Geometry check sheet. Reference: drawing and pictorial views, mm from the part's lowest x, y, z. A direction names the side the tool comes from. Coordinates: 2 decimals unless noted, no trailing zeros. Loops run counter-clockwise (first coordinate to the right, second up) from the corner with the lowest first, then second, coordinate; pieces in that order, holes last. Notation, with made-up numbers: (-10, 54.5) - (46, 54.5) arc R14 cw to (46, 78.5) - close; hole circle Ø2 at (54.5, 67). An arc over 180 degrees is marked (long way). One line per item, written item: value.
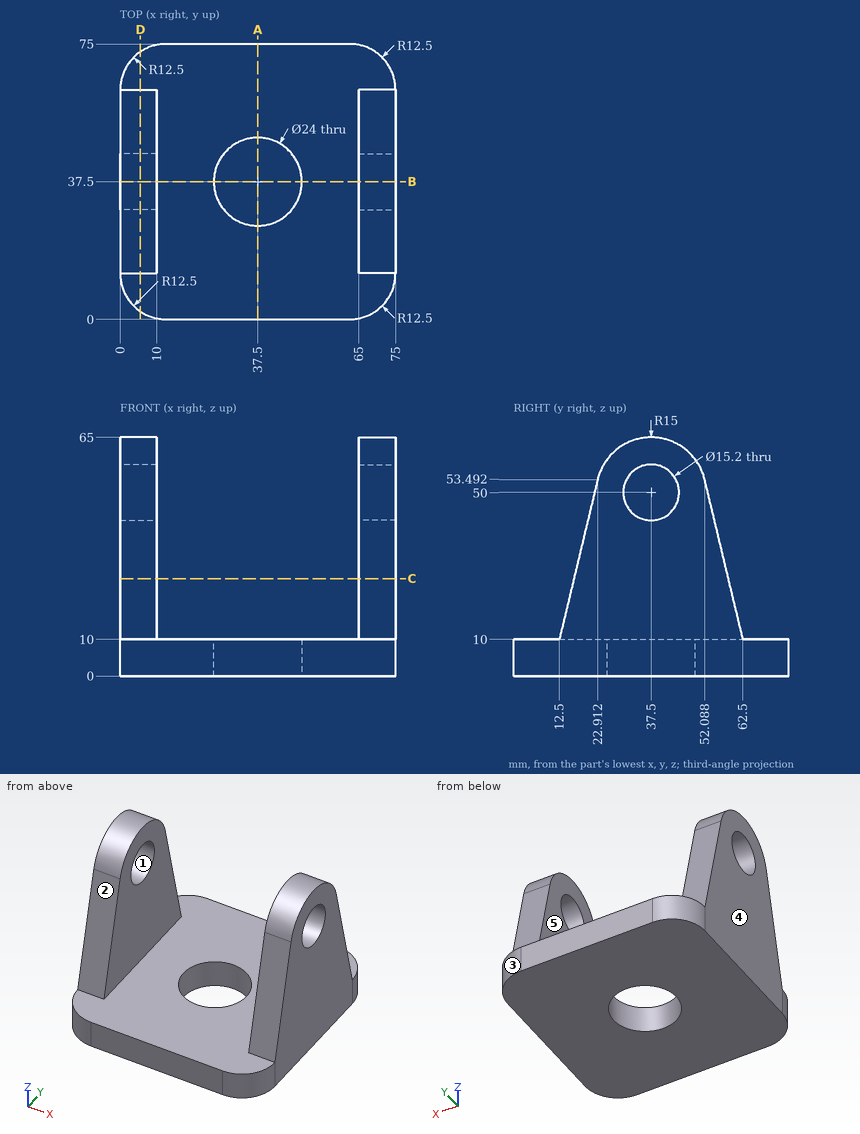
(1) Cross-section at B-B on y = 37.5. Record the cut outline in (x, z).
Reply:
outline: (0, 0) - (25.5, 0) - (25.5, 10) - (10, 10) - (10, 42.4) - (0, 42.4) - close; (0, 57.6) - (10, 57.6) - (10, 65) - (0, 65) - close; (49.5, 0) - (75, 0) - (75, 42.4) - (65, 42.4) - (65, 10) - (49.5, 10) - close; (65, 57.6) - (75, 57.6) - (75, 65) - (65, 65) - close
(2) Cross-section at C-C on z = 26.5. Record the cut outline in (x, y), and give its area (3 significant figures).
Reply:
outline: (0, 16.45) - (10, 16.45) - (10, 58.55) - (0, 58.55) - close; (65, 16.45) - (75, 16.45) - (75, 58.55) - (65, 58.55) - close
area: 842 mm2
(3) Cross-section at A-A on x = 37.5. Record the cut outline in (y, z).
Reply:
outline: (0, 0) - (25.5, 0) - (25.5, 10) - (0, 10) - close; (49.5, 0) - (75, 0) - (75, 10) - (49.5, 10) - close
(4) Go/stop test with flat-tipped pins: pin 1 Ø19 at (x, y) = (37.5, 37.5) entering from -Z; pin 2 Ø6 at (x, y) = (14.5, 50.5) entering from +Z; pin 3 Ø12 at (x, y) = (67, 53.5) entering from +Z; pin 4 Ø12 at (x, y) = (63.5, 44) entering from +Z. Record where each tip stops, or that it passes through.
Reply:
pin 1: through
pin 2: z = 10
pin 3: z = 61.18
pin 4: z = 64.98
(5) Release check for a two-part mould opening along Y. For the marked faces 1, 2 and 3 record: pulls with the +Y half, pulls with the -Y half, needs draft (parallel to the pull), parting line crosses it, or undercut.
Reply:
face 1: undercut
face 2: pulls with the -Y half
face 3: pulls with the +Y half
(6) Cross-section at D-D on x = 5.5. Record the cut outline in (y, z), and give its area (3 significant figures).
Reply:
outline: (2.14, 0) - (72.86, 0) - (72.86, 10) - (62.5, 10) - (52.09, 53.49) arc R15 ccw to (22.91, 53.49) - (12.5, 10) - (2.14, 10) - close; hole circle Ø15.2 at (37.5, 50)
area: 2,500 mm2
(7) Material ranges on probe 1 along X at (y, z) = (26.5, 23); probe 2 along Y at (x, z) = (37, 3), recorded low to high. Write a range as from..to.
Reply:
probe 1: 0..10, 65..75
probe 2: 0..25.51, 49.49..75
(8) Access from +Z, -Z, +X, -X, +Y, -Y to the whole of each face (thin tool, end or side, straight path). Record for the marked faces 4 and 5.
Reply:
face 4: +Z, -Z, -X, +Y, -Y
face 5: +Z, +Y, -Y
